from build123d import *

# Parameters (mm, degrees)
SKETCH1_R           = 3
BOSS_EXTRUDE1_DEPTH = 7


with BuildPart() as part:
    # Sketch1 → Boss-Extrude1 (new body)
    with BuildSketch(Plane(origin=(0, 0, 0), x_dir=(1, 0, 0), z_dir=(0, 1, 0))):
        Polygon((30, -77), (94.5, -77), (94.5, 77), (-85.39, 77), (-94.5, 77), (-94.5, -77), align=None)
        with Locations(Location((41, -60, 0), (0, 0, 270))):
            Circle(SKETCH1_R, mode=Mode.SUBTRACT)
        with Locations(Location((63, -60, 0), (0, 0, 270))):
            Circle(SKETCH1_R, mode=Mode.SUBTRACT)
        with Locations(Location((41, -21, 0), (0, 0, 270))):
            Circle(SKETCH1_R, mode=Mode.SUBTRACT)
        with Locations(Location((63, -21, 0), (0, 0, 270))):
            Circle(SKETCH1_R, mode=Mode.SUBTRACT)
        with Locations(Location((-74.39, 21, 0), (0, 0, 270))):
            Circle(SKETCH1_R, mode=Mode.SUBTRACT)
        with Locations(Location((-52.39, 21, 0), (0, 0, 270))):
            Circle(SKETCH1_R, mode=Mode.SUBTRACT)
        with Locations(Location((-74.39, 60, 0), (0, 0, 270))):
            Circle(SKETCH1_R, mode=Mode.SUBTRACT)
        with Locations(Location((-52.39, 60, 0), (0, 0, 270))):
            Circle(SKETCH1_R, mode=Mode.SUBTRACT)
    extrude(amount=BOSS_EXTRUDE1_DEPTH)


solid = part.part
Build history of the part. All positions in model axes, mm. Round coordinates to 2 decimals unless told otherwise and drop trailing zeros. Write each loop counter-clockwise with the first axis right and the second up, starting at its lowest first coordinate (ties: lowest second). Pieces come first, ordered by that corner, then holes. Notation, with made-up numbers: M 88.5,30 L 125.5,30 A23 cw 125.5,40 Z; hole C 68.25,16.5 d3. An arc over 180 degrees is marked long. Use CSV: the item, a comma, the result in double quotes.
1. Saw through at B-B (x = -74.39). Give the cut face in (y, z).
Reply:
outline,"M 0,-77 L 7,-77 L 7,-63 L 0,-63 Z; M 0,-57 L 7,-57 L 7,-24 L 0,-24 Z; M 0,-18 L 7,-18 L 7,77 L 0,77 Z"
2. Wall check: probe 1 along X at (y, z) = (4, -21); probe 2 along X at (y, z) = (3.5, 21). Give the ranges that are in metal, low to high. Write a range as from..to.
Reply:
probe 1,"x = -94.5..-77.39, -71.39..-55.39, -49.39..94.5"
probe 2,"x = -94.5..38, 44..60, 66..94.5"
3. Saw through at A-A (z = -60). Give the cut face in (x, y).
Reply:
outline,"M -94.5,0 L -77.39,0 L -77.39,7 L -94.5,7 Z; M -71.39,0 L -55.39,0 L -55.39,7 L -71.39,7 Z; M -49.39,0 L 94.5,0 L 94.5,7 L -49.39,7 Z"
4. Two-plate mould, pull along X, no slides. Class faces 1 (the face through (1, 3, -77)), 2 (the face through (-76.215, 3.451, -62.381)), 3 (the face through (94.5, 3, 1)): +X half, -X half, draft (parallel to the pull), parting line (faces both ways), or undercut.
Reply:
face 1,"draft"
face 2,"undercut"
face 3,"+X half"
